Input: part model. Units: mm. Frame: model coordinates. A direction names the side the tool comes from. Coordinates: 2 decimals unless noted, no trailing zeros. Order: outer loops, then holes, each group sorted by start corner. A loop starts at its lowest first (then second) coordinate and runs counter-clockwise, first axis right, second up. Notation, with made-up numbers: (29, -26.5) - (64, -26.5) arc R19 ccw to (64, -6.5) - close; hole circle Ø4 at (-18, 7.25). An arc over 180 degrees is marked (long way). Answer as CSV lines item,"result". Start each with the question number.
Item 1: Material intervals for line 1 along Z through (x, y) = (0.75, 0.75); line 2 along X through (y, z) = (-1, -7.25); line 3 along Y through (x, z) = (0.25, -7.25), sorted ascending.
Item 2: Draft query along X for faces 3 (the flat face through (1.25, 0, -8)), 4 (the flat face through (2, -2, -7)), 5 (the cylindrical face through (0, -2, -4)), 6 (the flat face through (0.63, -1.08, -8.11)). Return one class per face: +X half, -X half, draft (parallel to the pull), parting line (faces both ways), or undercut.
Item 3: Section B-B (z = -3). Output: boundary loops of the cut face in (x, y).
Item 4: Access query for faces 1 (the flat face through (0, 0, 0)), 2 (the flat face through (0.616, 1.088, -8.113)). Directions: +Z, -Z, +X, -X, +Y, -Y. A direction counts if a zero-diameter tool reaches every point of the face in a straight line with its end or side. Return the directions, or none.
Item 5: Section A-A (y = 0). Output: boundary loops of the cut face in (x, z).
Item 6: First-contact query: pin 1 (1 mm diameter, centred on y = 0.5, z = -5, fed in from +X); pin 2 (2 mm diameter, centred on y = -1, z = -8, fed in from -X); pin 3 (4 mm diameter, centred on x = -3, z = -4, fed in from +Y). Flat tips, straight axial feed; report the tip coordinate or a pass-through.
from build123d import *

# Parameters (mm, degrees)
CUT_EXTRUDE1_DEPTH = 1.8


with BuildPart() as part:
    # Sketch1 → Revolve1 (revolve)
    with BuildSketch(Plane(origin=(0, 0, 0), x_dir=(1, 0, 0), z_dir=(0, 1, 0))):
        with BuildLine():
            Line((0, 0), (-2, 0))
            Line((-2, 0), (-2, 7))
            Line((-2, 7), (-3.75, 7))
            ThreePointArc((-3.75, 7), (-3.328768227, 8.397047198), (-2, 9))
            Line((-2, 9), (0, 9))
            Line((0, 9), (0, 0))
        make_face()
    revolve(axis=Axis((0, 0, 0), (0, 0, -1)))

    # Sketch2 → Cut-Extrude1 (cut)
    with BuildSketch(Plane(origin=(0, 0, -9), x_dir=(-1, 0, 0), z_dir=(0, 0, -1))):
        Polygon((0, -1.443375673), (1.25, -0.721687836), (1.25, 0.721687836), (0, 1.443375673), (-1.25, 0.721687836), (-1.25, -0.721687836), align=None)
    extrude(amount=-CUT_EXTRUDE1_DEPTH, mode=Mode.SUBTRACT)


solid = part.part
Determined:
1,line 1,"z = -7.2 to 0"
1,line 2,"x = -3.63 to -0.77, 0.77 to 3.63"
1,line 3,"y = -3.76 to -1.3, 1.3 to 3.76"
2,face 3,"undercut"
2,face 4,"draft"
2,face 5,"parting line"
2,face 6,"undercut"
3,outline,"circle Ø4 at (0, 0)"
4,face 1,"+Z, +X, -X, +Y, -Y"
4,face 2,"-Z"
5,outline,"(-3.75, -7) arc R1.77 ccw to (-2, -9) - (-1.25, -9) - (-1.25, -7.2) - (1.25, -7.2) - (1.25, -9) - (2, -9) arc R1.77 ccw to (3.75, -7) - (2, -7) - (2, 0) - (-2, 0) - (-2, -7) - close"
6,pin 1,"stops at x = 2"
6,pin 2,"stops at x = -3.75"
6,pin 3,"stops at y = 1.73"
